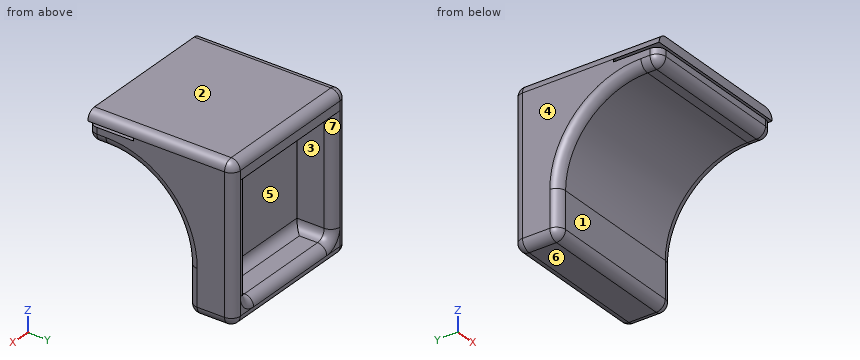
from build123d import *

# Parameters (mm, degrees)
F1_DEPTH  = 60
F2_DEPTH  = 85
F3_W      = 65
F3_H      = 20
F4_DEPTH  = 10
F5_W      = 65
F5_H      = 20
F6_DEPTH  = 10
F9_W      = 85
F9_H      = 25
F10_DEPTH = 1.5
F11_F1_R  = 5
F11_F2_R  = 5
F12_W     = 85
F12_H     = 60
F13_DEPTH = 70
F14_R     = 45
F15_R     = 4.99999
F16_R     = 4.99999
F17_W     = 85
F17_H     = 1.5
F18_DEPTH = 5
F19_W     = 85
F19_H     = 5
F20_DEPTH = 5
F21_W     = 5
F21_H     = 10
F22_DEPTH = 85
F23_R     = 4.99999


# Not quite as in the source:
# - a fillet or chamfer is up to 0.001 mm smaller than in the source, because OpenCascade refuses the exact size


with BuildPart() as f1:
    # F0 (on Top) → F1 (new body)
    with BuildSketch(Plane.XY):
        Polygon((-61.8206309527, 56.9930104911), (-61.8206309527, -28.0069895089), (23.1793690473, -28.0069895089), (23.1793690473, 56.9930104911), (13.1793690473, 56.9930104911), (13.1793690473, 36.9930104911), (-51.8206309527, 36.9930104911), (-51.8206309527, 56.9930104911), align=None)
    extrude(amount=F1_DEPTH)

    # F0 (on Top) → F2 (join)
    with BuildSketch(Plane.XY):
        Polygon((-61.8206309527, 56.9930104911), (-61.8206309527, -28.0069895089), (23.1793690473, -28.0069895089), (23.1793690473, 56.9930104911), (13.1793690473, 56.9930104911), (13.1793690473, 36.9930104911), (-51.8206309527, 36.9930104911), (-51.8206309527, 56.9930104911), align=None)
    extrude(amount=F2_DEPTH)

    # F3 (on face) → F4 (join)
    with BuildSketch(Plane.XY.offset(85)):
        with Locations((-19.3206309527, 46.9930104911)):
            Rectangle(F3_W, F3_H)
    extrude(amount=-F4_DEPTH)

    # F5 (on face) → F6 (join)
    with BuildSketch(Plane(origin=(0, 0, 0), x_dir=(1, 0, 0), z_dir=(0, 0, -1))):
        with Locations((-19.3206309527, -46.9930104911)):
            Rectangle(F5_W, F5_H)
    extrude(amount=-F6_DEPTH)

    # F9 (on offset) → F10 (cut)
    with BuildSketch(Plane.XY.offset(80)):
        with Locations((-19.3206309527, -15.5069895089)):
            Rectangle(F9_W, F9_H)
    extrude(amount=-F10_DEPTH, mode=Mode.SUBTRACT)

    # F11: fillet of radius 5 on 4 edges, made by hand

    # F11_f1
    f11_f1_edges = [f1.edges().sort_by_distance(p)[0] for p in [
        (13.1793690473, 46.9930104911, 10),
        (-19.3206309527, 36.9930104911, 10),
        (-51.8206309527, 46.9930104911, 10),
    ]]
    fillet(f11_f1_edges, radius=F11_F1_R)

    # F11_f2
    f11_f2_edges = [f1.edges().sort_by_distance(p)[0] for p in [
        (-19.3206309527, 56.9930104911, 10),
        (-50.3561648586, 56.9930104911, 11.4644660941),
        (11.7149029532, 56.9930104911, 11.4644660941),
    ]]
    fillet(f11_f2_edges, radius=F11_F2_R)

    # F12 (on face) → F13 (cut)
    with BuildSketch(Plane(origin=(0, 0, 0), x_dir=(1, 0, 0), z_dir=(0, 0, -1))):
        with Locations((-19.3206309527, -1.9930104911)):
            Rectangle(F12_W, F12_H)
    extrude(amount=-F13_DEPTH, mode=Mode.SUBTRACT)

    # F14
    f14_edges = [f1.edges().sort_by_distance(p)[0] for p in [
        (-19.320631, 31.99301, 70),
    ]]
    fillet(f14_edges, radius=F14_R)

    # F15 (radius 5 in the source; OpenCascade refuses exactly that, so slightly less here)
    f15_edges = [f1.edges().sort_by_distance(p)[0] for p in [
        (-19.320631, 56.99301, 0),
        (-61.820631, 56.99301, 42.5),
        (23.179369, 56.99301, 42.5),
        (-61.820631, 44.49301, 0),
        (23.179369, 44.49301, 0),
        (-19.320631, 31.99301, 0),
        (-61.820631, -20.50699, 70),
        (23.179369, 18.812816, 56.819805),
        (-61.820631, 31.99301, 12.5),
        (-61.820631, 18.812816, 56.819805),
        (-61.820631, 14.49301, 85),
        (23.179369, 31.99301, 12.5),
        (23.179369, -20.50699, 70),
        (-19.320631, 56.99301, 85),
        (23.179369, 14.49301, 85),
    ]]
    fillet(f15_edges, radius=F15_R)

    # F16 (radius 5 in the source; OpenCascade refuses exactly that, so slightly less here)
    f16_edges = [f1.edges().sort_by_distance(p)[0] for p in [
        (-19.320631, 51.99302, 0),
        (18.179379, 44.49301, 0),
        (-56.820641, 44.49301, 0),
        (-19.320631, 36.993, 0),
        (-19.320631, -28.00699, 70),
    ]]
    fillet(f16_edges, radius=F16_R)

    # F17 (on face) → F18 (cut)
    with BuildSketch(Plane.XZ.offset(3.0069895089)):
        with Locations((-19.3206309527, 79.25)):
            Rectangle(F17_W, F17_H)
    extrude(amount=-F18_DEPTH, mode=Mode.SUBTRACT)

    # F19 (on face) → F20 (cut)
    with BuildSketch(Plane.XZ.offset(28.0069895089)):
        with Locations((-19.3206309527, 82.5)):
            Rectangle(F19_W, F19_H)
    extrude(amount=-F20_DEPTH, mode=Mode.SUBTRACT)

    # F21 (on face) → F22 (cut)
    with BuildSketch(Plane(origin=(-61.8206309527, 0, 0), x_dir=(0, -1, 0), z_dir=(-1, 0, 0))):
        with Locations((25.5069895089, 73.5)):
            Rectangle(F21_W, F21_H)
    extrude(amount=-F22_DEPTH, mode=Mode.SUBTRACT)

    # F23 (radius 5 in the source; OpenCascade refuses exactly that, so slightly less here)
    f23_edges = [f1.edges().sort_by_distance(p)[0] for p in [
        (-19.320631, -23.00699, 70),
        (-61.820631, -23.00699, 76.749995),
        (-60.356168, -23.00699, 71.464463),
        (21.714906, -23.00699, 71.464463),
        (23.179369, -23.00699, 76.749995),
    ]]
    fillet(f23_edges, radius=F23_R)


solid = f1.part
Geometry check sheet. Reference: the model listing, model coordinates, mm. Face numbers are marked on the shaded views. A direction names the side the tool comes from. Give positions to 0.01 mm unless a question says otherwise; leave off trailing zeros. Order: outer loops, then holes, each group sorted by start corner. A loop starts at its lowest first (then second) coordinate and runs counter-clockwise, first axis right, second up.
1. Access from +Z, -Z, +X, -X, +Y, -Y to the whole of each face (thin tool, end or side, straight path). Record for the marked faces 1, 2 and 3.
Completed:
face 1: -Z, +X, -X, -Y
face 2: +Z, +X, -X, +Y, -Y
face 3: +Y
2. Scan lines: line 1 (X direction, y = 40.5, z = 28); line 2 (Z direction, x = -26, y = -16); line 3 (Y direction, x = 5, z = 19). Record each from-to range of solid material in increasing order.
Completed:
line 1: x = -61.82 to -51.82, 13.18 to 23.18
line 2: z = 70 to 78.5, 80 to 85
line 3: y = 31.99 to 36.99
3. Depth check by flat-ended pin: pin 1 (6 mm diameter, centred on x = -37.5, z = 36, fed in from -Y); pin 2 (22 mm diameter, centred on x = -3.5, z = 13, fed in from -Y); pin 3 (8 mm diameter, centred on x = -31.5, y = -2.5, fed in from -Z). Enter the tip coordinate at first touch or a pass-through.
Completed:
pin 1: stops at y = 29.76
pin 2: stops at y = 31.99
pin 3: stops at z = 67.6
4. Sectioned sample at A-A (y = 50.5). Record the boundary of the cut face in (x, z), then the cut area to 3 significant figures.
Completed:
outline: (-61.82, 5) arc R5 ccw to (-56.82, 0) - (18.18, 0) arc R5 ccw to (23.18, 5) - (23.18, 80) arc R5 ccw to (18.18, 85) - (-56.82, 85) arc R5 ccw to (-61.82, 80) - close; hole (-51.82, 15) arc R5 ccw to (-46.82, 10) - (8.18, 10) arc R5 ccw to (13.18, 15) - (13.18, 75) - (-51.82, 75) - close
area: 2,990 mm2
5. Draft check along X on the marked faces 4, 5, 6 and 7. Enter one of: pulls with the +X half, pulls with the -X half, needs draft (parallel to the pull), parting line crosses it, or undercut.
Completed:
face 4: pulls with the -X half
face 5: undercut
face 6: needs draft
face 7: undercut
